Autodesk Inventor part; units mm, degrees
ref_plane "Arbeitsebene1" through (27, 40, -27) normal (-0.7071, 0, -0.7071) x (0, -1, 0)
ref_plane "Arbeitsebene2" through (27, 40, 27) normal (0.7071, 0, -0.7071) x (0, -1, 0)
ref_plane "YZ Plane" through (0, 0, 0) normal (1, 0, 0) x (0, 1, 0)
sketch "Skizze1" plane through (0, 0, 0) normal (0, 1, 0) x (-1, 0, 0)
  line L0 (-27, 27) -> (27, 27)
  line L1 (27, 27) -> (27, -27)
  line L2 (27, -27) -> (-27, -27)
  line L3 (-27, -27) -> (-27, 27)
  line L4 (-27, 27) -> (27, -27) construction
  line L5 (27, 27) -> (-27, -27) construction
  point P0 (0, 0)
  dimension "d0" = 54
  dimension "d1" = 54
extrude "Extrusion1" add sketch "Skizze1" along normal blind 40
sketch "Skizze2" plane through (0, 40, 0) normal (0, 1, 0) x (1, 0, 0)
  line L0 (23, -23) -> (-23, -23)
  line L1 (-23, -23) -> (-23, 23)
  line L2 (-23, 23) -> (23, 23)
  line L3 (23, 23) -> (23, -23)
  line L4 (23, -23) -> (-23, 23) construction
  line L5 (-23, -23) -> (23, 23) construction
  line L6 (-27, -27) -> (27, -27)
  line L7 (27, -27) -> (27, 27)
  line L8 (27, 27) -> (-27, 27)
  line L9 (-27, 27) -> (-27, -27)
  point P0 (0, 0)
  dimension "d4" = 4
  dimension "d5" = 4
extrude "Extrusion2" cut sketch "Skizze2" against normal blind 35 contours L0 L1 L2 L3
fillet "Rundung1" radius 4 4 edges at (-23, 22.5, -23) (23, 22.5, -23) (-23, 22.5, 23) (23, 22.5, 23)
sketch "Skizze3" plane through (0, 0, 0) normal (0, -1, 0) x (1, 0, 0)
  line L0 (-18, 18) -> (18, 18)
  line L1 (18, 18) -> (18, -18)
  line L2 (18, -18) -> (-18, -18)
  line L3 (-18, -18) -> (-18, 18)
  line L4 (-18, 18) -> (18, -18) construction
  line L5 (18, 18) -> (-18, -18) construction
  line L6 (18, 0) -> (-18, 0) construction
  line L7 (0, 18) -> (0, -18) construction
  point P0 (0, 0)
  dimension "d9" = 36
  dimension "d10" = 36
hole "Bohrung1" at (18, 0, 18) at (18, 0, 0) at (18, 0, -18) at (0, 0, -18) at (-18, 0, -18) at (-18, 0, 0) at (-18, 0, 18) at (0, 0, 18) direction (0, 1, 0) diameter 3.4 end through all
sketch "Skizze5" plane through (27, 0, 27) normal (1, 0, 0) x (0, 0, -1)
  line L0 (9.5, 7.25) -> (44.5, 7.25)
  line L1 (44.5, 7.25) -> (44.5, 34.75)
  line L2 (44.5, 34.75) -> (9.5, 34.75)
  line L3 (9.5, 34.75) -> (9.5, 7.25)
  line L4 (9.5, 7.25) -> (44.5, 34.75) construction
  line L5 (44.5, 7.25) -> (9.5, 34.75) construction
  line L6 (54, 0) -> (0, 0)
  line L7 (54, 0) -> (54, 40)
  line L8 (0, 40) -> (54, 40)
  line L9 (0, 0) -> (0, 40)
  point P0 (27, 0)
  point P1 (27, 21)
  dimension "d18" = 9.5
  dimension "d21" = 35
  dimension "d29" = 27.5
  dimension "d30" = 54
  dimension "d46" = 21
  dimension "d47" = 27
hole "Bohrung2" at (27, 34.75, 17.5) at (27, 21, 0) at (27, 34.75, -17.5) at (27, 7.25, -17.5) at (27, 7.25, 17.5) direction (-1, 0, 0) diameter 2.459 depth 8.8 tip angle 118
ref_plane "Arbeitsebene1" through (27, 40, -27) normal (-0.7071, 0, -0.7071) x (0, -1, 0)
mirror "Spiegeln1" about plane through (27, 40, -27) normal (-0.7071, 0, -0.7071) of "Bohrung2"
ref_plane "Arbeitsebene2" through (27, 40, 27) normal (0.7071, 0, -0.7071) x (0, -1, 0)
mirror "Spiegeln2" about plane through (27, 40, 27) normal (0.7071, 0, -0.7071) of "Bohrung2", "Spiegeln1"
chamfer "Fase3" distance 2 angle 45 4 edges at (27, 20, 27) (27, 20, -27) (-27, 20, -27) (-27, 20, 27)
equation "\"d18\" = -0.5 * d21 + 0.5 * d30"
properties part number "cube_square_tube" material "Aluminium 6061"
Model file for the job. Use its own axes, mm. A direction names the side the tool comes from. Give positions to 0.01 mm unless a question says otherwise; leave off trailing zeros. Write each loop counter-clockwise with the first axis right and the second up, starting at its lowest first coordinate (ties: lowest second). Pieces come first, ordered by that corner, then holes. Notation, with made-up numbers: (24, 84) -> (48, 84) arc R18 cw to (48, 119) -> close; hole circle Ø4 at (64, -27.75). An arc over 180 degrees is marked (long way). Write item = value, one per line.
(1) Slice it at B-B, the plane y = 27.5. Give the cut face in (x, z), then the cut area to 3 significant figures.
Determined:
outline = (-27, -25) -> (-25, -27) -> (25, -27) -> (27, -25) -> (27, 25) -> (25, 27) -> (-25, 27) -> (-27, 25) -> close; hole (-23, -19) arc R4 ccw to (-19, -23) -> (19, -23) arc R4 ccw to (23, -19) -> (23, 19) arc R4 ccw to (19, 23) -> (-19, 23) arc R4 ccw to (-23, 19) -> close
area = 806 mm2
(2) Slice it at A-A, the plane z = 0. Give the cut face in (x, y).
Determined:
outline = (-27, 0) -> (-19.7, 0) -> (-19.7, 5) -> (-23, 5) -> (-23, 19.77) -> (-27, 19.77) -> close; (-27, 22.23) -> (-23, 22.23) -> (-23, 40) -> (-27, 40) -> close; (-16.3, 0) -> (16.3, 0) -> (16.3, 5) -> (-16.3, 5) -> close; (19.7, 0) -> (27, 0) -> (27, 19.77) -> (23, 19.77) -> (23, 5) -> (19.7, 5) -> close; (23, 22.23) -> (27, 22.23) -> (27, 40) -> (23, 40) -> close
(3) Probe line 1 along Z through (x, y) = (24.5, 7.25); line 2 along X through (y, z) = (2, 0). List the from-to ranges inside material, lowest first.
Determined:
line_1 = -27 to -18.73, -16.27 to 16.27, 18.73 to 27
line_2 = -27 to -19.7, -16.3 to 16.3, 19.7 to 27
(4) Mould opens along Z. For faces 1 (the face through (24.972, 33.713, 16.839)), 2 (the face through (0, 23, 23)), 3 (the face through (18.161, 35.787, -24.972)), 4 (the face through (26, 20, -26)) say: released by +Z, released by -Z, zero draft, split by the parting line, or undercut.
Determined:
face_1 = undercut
face_2 = undercut
face_3 = zero draft
face_4 = released by -Z
(5) Tool access for faces 5 (the face through (23, 23, 0)), 6 (the face through (-24.972, 33.713, -16.839)): list every direction of +Z, -Z, +X, -X, +Y, -Y with a clear straight run to the whole face (end or side of a thin tool).
Determined:
face_5 = +Y
face_6 = +X, -X
(6) Slice it at C-C, the plane x = 0. Give the cut face in (y, z), then the cut area to 3 significant figures.
Determined:
outline = (0, -27) -> (19.77, -27) -> (19.77, -23) -> (5, -23) -> (5, -19.7) -> (0, -19.7) -> close; (0, -16.3) -> (5, -16.3) -> (5, 16.3) -> (0, 16.3) -> close; (0, 19.7) -> (5, 19.7) -> (5, 23) -> (19.77, 23) -> (19.77, 27) -> (0, 27) -> close; (22.23, -27) -> (40, -27) -> (40, -23) -> (22.23, -23) -> close; (22.23, 23) -> (40, 23) -> (40, 27) -> (22.23, 27) -> close
area = 496 mm2
(7) Flat gauge pins, fed straight in: P1, Ø2, axis at x = 9.5, z = 19.5, coming from the +Y side; P2, Ø2, axis at y = 21, z = 0, coming from the +X side. Where does each tip first touch, or does it go through?
Determined:
P1 = 5
P2 = through
(8) Slice it at D-D, the plane y = 21. Give the number of separate pieces and of enclosed holes in the cut face, then the cut area to 3 significant figures.
Determined:
separate_pieces = 4
enclosed_holes = 0
area = 766 mm2
